```python
from build123d import *

# Parameters (mm, degrees)
SKETCH1_W                = 20.574
SKETCH1_H                = 44.196
BOSS_EXTRUDE1_DEPTH      = 1.397
SHELL1_T                 = -0.508
CUT_EXTRUDE1_DEPTH       = 25.415068749
CUT_EXTRUDE1_DEPTH_BACK  = 25.415068749
CUT_EXTRUDE2_DEPTH       = 25.415068749
CUT_EXTRUDE2_DEPTH_BACK  = 25.415068749
SKETCH5_W                = 2.286
SKETCH5_H                = 5.08
BOSS_EXTRUDE2_DEPTH      = 0.508
BOSS_EXTRUDE3_DEPTH      = 5.842
BOSS_EXTRUDE3_DEPTH_BACK = 0.635
SKETCH6_W                = 6.35
SKETCH6_H                = 1.778
BOSS_EXTRUDE4_DEPTH      = 3.175
SKETCH8_R                = 0.381
CUT_EXTRUDE3_DEPTH       = 31.873801871
FILLET1_R                = 0.381
CIRPATTERN1_START        = -3.175
CIRPATTERN1_DEPTH        = 6.35
CUT_EXTRUDE4_DEPTH       = 31.853319649
CUT_EXTRUDE4_DEPTH_BACK  = 31.853319649
BOSS_EXTRUDE5_DEPTH      = 1.397
BOSS_EXTRUDE6_REACH      = 32.853
SHELL2_START             = -7.869211645
SHELL2_OUTLINE_W         = 5.08
SHELL2_OUTLINE_H         = 0.889
SHELL2_DEPTH             = 0.762
FILLET2_R                = 0.381
FILLET6_R                = 0.127


# Read off the part's stored shape, not the designer's step: CirPattern1, Shell2
with BuildPart() as part:
    # Sketch1 → Boss-Extrude1 (new, symmetric)
    with BuildSketch(Plane(origin=(0, 0, 0), x_dir=(1, 0, 0), z_dir=(0, 1, 0))):
        Rectangle(SKETCH1_W, SKETCH1_H)
    extrude(amount=BOSS_EXTRUDE1_DEPTH, both=True)

    # Shell1
    shell1_openings = [part.faces().sort_by_distance(p)[0] for p in [
        (0, 1.397, 0),
    ]]
    offset(amount=SHELL1_T, openings=shell1_openings, kind=Kind.INTERSECTION)

    # Sketch3 → Cut-Extrude1 (cut, two sides: drawn at the far end of the back side and taken through both)
    with BuildSketch(Plane(origin=(0, 0, 0), x_dir=(1, 0, 0), z_dir=(0, 1, 0)).offset(-CUT_EXTRUDE1_DEPTH_BACK)):
        Polygon((10.287, 22.098), (-9.779, -0.254), (-9.779, 22.098), align=None)
    extrude(amount=CUT_EXTRUDE1_DEPTH + CUT_EXTRUDE1_DEPTH_BACK, mode=Mode.SUBTRACT)

    # Sketch4 → Cut-Extrude2 (cut, two sides: drawn at the far end of the back side and taken through both)
    with BuildSketch(Plane(origin=(0, 0, 0), x_dir=(1, 0, 0), z_dir=(0, 1, 0)).offset(-CUT_EXTRUDE2_DEPTH_BACK)):
        with BuildLine():
            Line((-10.287, -22.098), (10.287, -22.098))
            Line((10.287, -22.098), (10.287, -15.748))
            Line((10.287, -15.748), (5.207, -15.748))
            Line((5.207, -15.748), (3.864134037, -14.80771513))
            ThreePointArc((3.864134037, -14.80771513), (3.740583181, -14.762746296), (3.611100584, -14.785577571))
            Line((3.611100584, -14.785577571), (0.917342395, -16.041697644))
            ThreePointArc((0.917342395, -16.041697644), (0.786005508, -16.185026705), (0.794485256, -16.37924486))
            Line((0.794485256, -16.37924486), (0.901830294, -16.609447038))
            Line((0.901830294, -16.609447038), (-9.779, -21.59))
            Line((-9.779, -21.59), (-10.287, -21.59))
            Line((-10.287, -21.59), (-10.287, -22.098))
        make_face()
    extrude(amount=CUT_EXTRUDE2_DEPTH + CUT_EXTRUDE2_DEPTH_BACK, mode=Mode.SUBTRACT)

    # Sketch5 → Boss-Extrude2 (add)
    with BuildSketch(Plane.ZY.offset(10.287)):
        with Locations((-23.241, 0)):
            Rectangle(SKETCH5_W, SKETCH5_H)
    extrude(amount=-BOSS_EXTRUDE2_DEPTH)

    # Sketch6 → Boss-Extrude3 (add, two sides: drawn at the far end of the back side and taken through both)
    with BuildSketch(Plane.ZY.offset(10.287).offset(-BOSS_EXTRUDE3_DEPTH_BACK)):
        with Locations((-16.129, 0)):
            Rectangle(SKETCH6_W, SKETCH6_H)
    extrude(amount=BOSS_EXTRUDE3_DEPTH + BOSS_EXTRUDE3_DEPTH_BACK)

    # Sketch7 → Boss-Extrude4 (add, symmetric)
    with BuildSketch(Plane(origin=(0, 0, 0), x_dir=(1, 0, 0), z_dir=(0, 1, 0))):
        with BuildLine():
            Line((-16.129, 11.049), (-16.129, 21.209))
            ThreePointArc((-16.129, 21.209), (-18.669, 16.129), (-16.129, 11.049))
        make_face()
    extrude(amount=BOSS_EXTRUDE4_DEPTH, both=True)

    # Sketch8 → Cut-Extrude3 (cut, symmetric)
    with BuildSketch(Plane(origin=(0, 0, 0), x_dir=(1, 0, 0), z_dir=(0, 1, 0))):
        with Locations((-17.145, 20.25601151)):
            Circle(SKETCH8_R)
    extrude(amount=CUT_EXTRUDE3_DEPTH, both=True, mode=Mode.SUBTRACT)

    # Fillet1
    # the kernel refuses this fillet: 0.381 mm, written as the material it takes off along each edge
    with BuildSketch(Plane(origin=(-16.129, -5.314598451, -21.209), x_dir=(0, 0, 1), z_dir=(0, 1, 0))) as fillet1_piece_1:
        with BuildLine():
            CenterArc((0.829767065, -0.381), FILLET1_R, 90, 134.597956661)
            ThreePointArc((0.558475601, -0.648510638), (0.268299759, -0.333674793), (0, 0))
            Line((0, 0), (0.829767065, 0))
        make_face()
    extrude(amount=10.629196903, mode=Mode.SUBTRACT)
    with BuildSketch(Plane(origin=(-16.888803964, -3.924719523, -20.538012558), x_dir=(0.5312847358041962, 0, 0.8471933247502991), z_dir=(0, 1, 0))) as fillet1_piece_2:
        with BuildLine():
            CenterArc((0.308389086, 0.366870424), FILLET1_R, 191.227508383, 63.119725462)
            ThreePointArc((-0.065319255, 0.292687706), (-0.034387693, 0.1459582), (0, 0))
            ThreePointArc((0, 0), (0.102796362, 0.014129576), (0.205592724, 0))
        make_face()
    extrude(amount=7.849439047, mode=Mode.SUBTRACT)
    with BuildSketch(Plane(origin=(-17.383822436, -3.924719523, -19.95915322), x_dir=(0.919383333537804, 0, 0.39336279185112943), z_dir=(0, 1, 0))) as fillet1_piece_3:
        with BuildLine():
            CenterArc((0.308389086, -0.366870424), FILLET1_R, 105.652766155, 63.119725462)
            ThreePointArc((-0.065319255, -0.292687706), (-0.034387693, -0.1459582), (0, 0))
            ThreePointArc((0, 0), (0.102796362, -0.014129576), (0.205592724, 0))
        make_face()
    extrude(amount=7.849439047, mode=Mode.SUBTRACT)

    # CirPattern1 outline → CirPattern1 (cut)
    with BuildSketch(Plane(origin=(0, 0, 0), x_dir=(1, 0, 0), z_dir=(0, 1, 0)).offset(CIRPATTERN1_START)):
        with BuildLine():
            ThreePointArc((-16.777510638, 11.607475601), (-16.809726428, 11.745008607), (-16.789621511, 11.884826264))
            ThreePointArc((-16.789621511, 11.884826264), (-16.855265692, 12.249273725), (-17.19948569, 12.38581567))
            ThreePointArc((-17.19948569, 12.38581567), (-17.404514793, 12.415873831), (-17.563486704, 12.548796206))
            ThreePointArc((-17.563486704, 12.548796206), (-17.193275379, 12.059117997), (-16.777510638, 11.607475601))
        make_face()
        with BuildLine():
            ThreePointArc((-16.129, 11.878767065), (-16.36296353, 11.527282675), (-16.777510638, 11.607475601))
            ThreePointArc((-16.777510638, 11.607475601), (-16.462674793, 11.317299759), (-16.129, 11.049))
            Line((-16.129, 11.049), (-16.129, 11.878767065))
        make_face()
        with BuildLine():
            ThreePointArc((-17.633655181, 19.604189248), (-17.975088939, 19.015374527), (-18.251537846, 18.393397205))
            ThreePointArc((-18.251537846, 18.393397205), (-18.127780644, 18.559603646), (-17.935337257, 18.63645395))
            ThreePointArc((-17.935337257, 18.63645395), (-17.635723603, 18.842192055), (-17.644932405, 19.20552621))
            ThreePointArc((-17.644932405, 19.20552621), (-17.695623525, 19.406451162), (-17.633655181, 19.604189248))
        make_face()
        with BuildLine():
            ThreePointArc((-18.298077653, 18.26748788), (-18.492621503, 17.615236028), (-18.616234382, 16.945908274))
            ThreePointArc((-18.616234382, 16.945908274), (-18.534696725, 17.136412963), (-18.365510912, 17.256064903))
            ThreePointArc((-18.365510912, 17.256064903), (-18.122204213, 17.526061867), (-18.215977249, 17.877207318))
            ThreePointArc((-18.215977249, 17.877207318), (-18.312172768, 18.060747091), (-18.298077653, 18.26748788))
        make_face()
        with BuildLine():
            ThreePointArc((-18.632095343, 16.812613331), (-18.66899876, 16.132967891), (-18.632944744, 15.453276862))
            ThreePointArc((-18.632944744, 15.453276862), (-18.598132415, 15.657552479), (-18.46155341, 15.81339407))
            ThreePointArc((-18.46155341, 15.81339407), (-18.287998835, 16.132729817), (-18.461154191, 16.452282211))
            ThreePointArc((-18.461154191, 16.452282211), (-18.59753833, 16.608294367), (-18.632095343, 16.812613331))
        make_face()
        with BuildLine():
            ThreePointArc((-18.617250379, 15.319962201), (-18.494474074, 14.650480486), (-18.300745514, 13.997986017))
            ThreePointArc((-18.300745514, 13.997986017), (-18.314582249, 14.20474426), (-18.218157429, 14.388163671))
            ThreePointArc((-18.218157429, 14.388163671), (-18.12394563, 14.739191657), (-18.366914716, 15.009492478))
            ThreePointArc((-18.366914716, 15.009492478), (-18.535950864, 15.129355761), (-18.617250379, 15.319962201))
        make_face()
        with BuildLine():
            ThreePointArc((-18.254363096, 13.872018629), (-17.978691709, 13.249696306), (-17.637994075, 12.660455345))
            ThreePointArc((-17.637994075, 12.660455345), (-17.699715253, 12.85827072), (-17.64877307, 13.059132165))
            ThreePointArc((-17.64877307, 13.059132165), (-17.639110206, 13.422454528), (-17.93846651, 13.628566908))
            ThreePointArc((-17.93846651, 13.628566908), (-18.130813704, 13.705657654), (-18.254363096, 13.872018629))
        make_face()
    extrude(amount=CIRPATTERN1_DEPTH, mode=Mode.SUBTRACT)

    # Sketch9 → Cut-Extrude4 (cut, two sides: drawn at the far end of the back side and taken through both)
    with BuildSketch(Plane(origin=(0, 0, 0), x_dir=(1, 0, 0), z_dir=(0, 1, 0)).offset(-CUT_EXTRUDE4_DEPTH_BACK)):
        with BuildLine():
            Line((-8.001, -11.938), (-10.287, -11.938))
            Line((-10.287, -11.938), (-10.287, -13.462))
            Line((-10.287, -13.462), (-8.001, -13.462))
            ThreePointArc((-8.001, -13.462), (-7.239, -12.7), (-8.001, -11.938))
        make_face()
        with BuildLine():
            Line((-8.001, -9.144), (-10.287, -9.144))
            Line((-10.287, -9.144), (-10.287, -3.048))
            Line((-10.287, -3.048), (-7.015482933, -7.0729656))
            ThreePointArc((-7.015482933, -7.0729656), (-6.854218921, -8.419704275), (-8.001, -9.144))
        make_face()
    extrude(amount=CUT_EXTRUDE4_DEPTH + CUT_EXTRUDE4_DEPTH_BACK, mode=Mode.SUBTRACT)

    # Sketch10 → Boss-Extrude5 (add)
    with BuildSketch(Plane(origin=(0, 0, 0), x_dir=(1, 0, 0), z_dir=(0, 1, 0))):
        with BuildLine():
            Line((-10.287, -3.048), (-9.779, -3.672995219))
            ThreePointArc((-9.779, -3.672995219), (-9.713577615, -4.485652185), (-9.518995533, -5.277377672))
            ThreePointArc((-9.518995533, -5.277377672), (-9.690211017, -5.601822413), (-10.00699519, -5.416817226))
            ThreePointArc((-10.00699519, -5.416817226), (-10.216755971, -4.240654366), (-10.287, -3.048))
        make_face()
    extrude(amount=BOSS_EXTRUDE5_DEPTH)

    # Boss-Extrude6: up to this face of the body (flat: up to its plane)
    boss_extrude6_end = Plane(part.part.faces().sort_by_distance((1.063267264, -1.397, 2.310847226))[0])
    # Sketch11 → Boss-Extrude6 (add, up to the picked face)
    with BuildSketch(Plane(origin=(0, 0, 0), x_dir=(1, 0, 0), z_dir=(0, 1, 0)), mode=Mode.PRIVATE) as boss_extrude6_sk1:
        Polygon((-1.696795769, 8.748961675), (-2.641846577, 9.59735956), (0.751744961, 13.377562792), (1.696795769, 12.529164907), align=None)
    boss_extrude6_tool1 = split(extrude(boss_extrude6_sk1.sketch, amount=-BOSS_EXTRUDE6_REACH, mode=Mode.PRIVATE), bisect_by=boss_extrude6_end, keep=Keep.BOTH, mode=Mode.PRIVATE)
    add(boss_extrude6_tool1.solids().sort_by(Axis((-0.472525, 0, -11.063262), (0, -1, 0)))[0])

    # Shell2 outline → Shell2 (cut)
    with BuildSketch(Plane(origin=(0, 0, 0), x_dir=(0.668029830269147, 0, -0.7441344944770231), z_dir=(0.7441344944770231, 0, 0.6680298302691471)).offset(SHELL2_START)):
        with Locations((7.916893984, -0.4445)):
            Rectangle(SHELL2_OUTLINE_W, SHELL2_OUTLINE_H)
    extrude(amount=SHELL2_DEPTH, mode=Mode.SUBTRACT)

    # Fillet2
    fillet2_edges = [part.edges().sort_by_distance(p)[0] for p in [
        (-16.129, 0, -19.304),
        (-16.129, -0.889, -16.129),
        (-16.129, 0, -12.954),
        (-16.129, 0.889, -16.129),
        (-9.779, -0.889, 1.963497609),
        (-9.779, -0.889, 10.541),
        (-9.779, -0.889, 17.526),
        (-10.287, -1.397, 10.541),
        (-10.287, -1.397, 17.526),
        (0.940755122, 0, -13.207883215),
        (-2.452836415, 0, -9.427679983),
        (-0.945050808, -1.397, -11.487461176),
        (-0.567030485, -0.889, -11.148102022),
        (9.779, -0.889, -2.892063291),
        (10.287, -1.397, -3.175),
        (-10.287, -1.397, -9.525),
    ]]
    fillet(fillet2_edges, radius=FILLET2_R)

    # Fillet6
    fillet6_edges = [part.edges().sort_by_distance(p)[0] for p in [
        (-9.7155, -0.889, -19.304),
        (-9.7155, 0.889, -19.304),
        (-9.7155, 0.889, -12.954),
        (-9.7155, -0.889, -12.954),
    ]]
    fillet(fillet6_edges, radius=FILLET6_R)


solid = part.part
```
The listing builds one solid part. Answer for the finished solid, in the listing's coordinates (mm). A direction names the side the tool comes from. Coordinates: 2 decimals unless noted, no trailing zeros. Loops run counter-clockwise (first coordinate to the right, second up) from the corner with the lowest first, then second, coordinate; pieces in that order, holes last. Notation, with made-up numbers: M -12.5,82 L 15.5,82 A23 ccw 15.5,91 Z; hole C -8,-20.75 d8. An arc over 180 degrees is marked long. Answer as a JSON object with one key per item and string values. Group by question number.
Item 1: Which of the six approach directions +Z, -Z, +X, -X, +Y, -Y give full straight-line access (tool end or side, diameter ignored) to faces 1 (the face through (9.779, 0, -3)), 2 (the face through (-9.779, 0, 17)), 3 (the face through (-9.652, 0, -16)), 4 (the face through (-10, -1, 9.144)), 5 (the face through (-13, -0.889, -16))?
Item 2: Section D-D (x = 4.5) is taken. Write down the section's boundary in (y, z), and give its area (3 significant figures).
Item 3: Section B-B (z = -2) is taken. Write down the section's boundary in (x, y), and give its area (3 significant figures).
Item 4: Each of these flat-tipped pins is pushed along its axis until it touches: P1, Ø4.5, axis at x = -12, z = -17.5, coming from the +Y side; P2, Ø1, axis at y = -1.5, z = 16.5, coming from the -X side; P3, Ø1.5, axis at y = 1, z = -11, coming from the -X side. Where does it stop, or does it pass through?
Item 5: Consider L1, parallel to X at y = 1.25, z = 10.5; L2, parallel to Y at x = 4, z = -7; L3, parallel to X at y = -0.75, z = -12.5. Determine where each line is inside the solid, lowest interval first.
Item 6: Section C-C (z = 12.7) is taken. Write down the section's boundary in (x, y).
Item 7: Determine the mould class of faces 6 (the face through (-10.215, 0.689, 4.257)), 7 (the face through (4.54, -1.15, 15.28)), 8 (the face through (-0.84, -1.282, -11.441)), 9 (the face through (1, -0.889, 2)) for opening direction Z: +Z half, -Z half, draft (parallel to the pull), parting line (faces both ways), or undercut.
Solved:
{
 "1": {"face 1": "+Z, -Z, +Y", "face 2": "+Z, +Y", "face 3": "-Z, +Y, -Y", "face 4": "-X, +Y, -Y", "face 5": "+Z, -Z, -Y"},
 "2": {"outline": "M -1.4,-15.65 L -0.89,-15.65 L -0.89,15.25 L -1.4,15.25 Z", "area": "15.7 mm2"},
 "3": {"outline": "M -10.29,-1.02 A0.38 ccw -9.91,-1.4 L -9.78,-1.4 L -9.78,1.4 L -10.29,1.4 Z; M -7.76,-1.4 L 9.91,-1.4 A0.38 ccw 10.29,-1.02 L 10.29,1.4 L 9.78,1.4 L 9.78,-0.51 A0.38 cw 9.4,-0.89 L -7.76,-0.89 Z", "area": "11.7 mm2"},
 "4": {"P1": "stops at y = 1.4", "P2": "stops at x = -10.29", "P3": "stops at x = -16.81"},
 "5": {"L1": "x = -10.29 to -9.78, 9.78 to 10.29", "L2": "y = -1.4 to -0.89", "L3": "x = -17.52 to -16.13, -10.29 to -9.78, -0.04 to 0.76, 9.69 to 10.29"},
 "6": {"outline": "M -7.24,-1.4 L 9.91,-1.4 A0.38 ccw 10.29,-1.02 L 10.29,1.4 L 9.78,1.4 L 9.78,-0.51 A0.38 cw 9.4,-0.89 L -7.24,-0.89 Z"},
 "7": {"face 6": "undercut", "face 7": "+Z half", "face 8": "-Z half", "face 9": "draft"}
}
